Input: part model. Units: mm. Frame: model coordinates. Face numbers are marked on the shaded views. A direction names the side the tool comes from. Round coordinates to 2 decimals unless told otherwise and drop trailing zeros. Loops run counter-clockwise (first coordinate to the right, second up) from the corner with the lowest first, then second, coordinate; pieces in that order, holes last. Notation, with made-up numbers: (25.25, -24.75) -> (62.25, -24.75) arc R9 ccw to (62.25, -15.75) -> close; hole circle Ø5 at (-11, -16). An arc over 180 degrees is marked (long way). Answer as a JSON object with one key per item and string values.
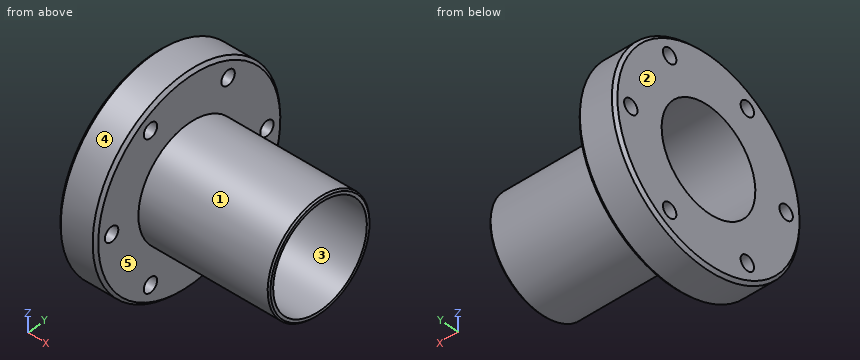
```python
from build123d import *

# Parameters (mm, degrees)
HOLE_WIZARD_M6_1_D       = 5
PATTERN_CIRCULAR_1_COUNT = 6
CHAMFER_1_SIZE           = 1
CHAMFER_2_SIZE           = 1
CHAMFER_3_SIZE           = 0.5


with BuildPart() as part:
    # 스케치1 → 회전1 (revolve)
    with BuildSketch(Plane.XY, mode=Mode.PRIVATE) as revolve_1_sk:
        Polygon((0, 17.5), (0, 35), (13, 35), (13, 19), (58, 19), (58, 17.5), align=None)
    revolve(revolve_1_sk.sketch.rotate(Axis((0, 0, 0), (1, 0, 0)), 90), axis=Axis((0, 0, 0), (1, 0, 0)))

    # M6 나사 구멍1 (through all)
    with Locations(Plane.ZY):
        with Locations((0, 29)):
            hole_wizard_m6_1 = Hole(HOLE_WIZARD_M6_1_D / 2)

    # 원형 패턴1: M6 나사 구멍1 ×6 about axis
    pattern_circular_1_axis = Axis((0, 0, 0), (1, 0, 0))
    for i in range(1, PATTERN_CIRCULAR_1_COUNT):
        add(hole_wizard_m6_1.rotate(pattern_circular_1_axis, i * 360 / PATTERN_CIRCULAR_1_COUNT), mode=Mode.SUBTRACT)

    # 모따기1
    chamfer_1_edges = [part.edges().sort_by_distance(p)[0] for p in [
        (0, 0, -35),
    ]]
    chamfer(chamfer_1_edges, length=CHAMFER_1_SIZE)

    # 모따기2
    chamfer_2_edges = [part.edges().sort_by_distance(p)[0] for p in [
        (13, 0, -35),
    ]]
    chamfer(chamfer_2_edges, length=CHAMFER_2_SIZE)

    # 모따기3
    chamfer_3_edges = [part.edges().sort_by_distance(p)[0] for p in [
        (58, 0, -19),
    ]]
    chamfer(chamfer_3_edges, length=CHAMFER_3_SIZE)


solid = part.part
```
1) Reachability of the marked faces 4 and 5 from +Z, -Z, +X, -X, +Y, -Y: full face, straight path, thin tool, end or side. Return the list, or none.
Output:
{"face 4": "+X, -X", "face 5": "+X"}
2) Ray query, probe 1 along Y at (x, z) = (4, 0); probe 2 along Z at (x, y) = (6, 14); probe 3 along X at (y, z) = (21.5, 10). Return the intervals inside material, ascending.
Output:
{"probe 1": "y = -35 to -31.5, -26.5 to -17.5, 17.5 to 26.5, 31.5 to 35", "probe 2": "z = -32.08 to -27.56, -22.67 to -10.5, 10.5 to 22.67, 27.56 to 32.08", "probe 3": "x = 0 to 13"}
3) Contact query for flat-ended pins moving along their axis: P1, Ø6, axis at x = 38, z = -8, coming from the -Y side; P2, Ø6.5, axis at y = -29, z = 0, coming from the +X side; P3, Ø12, axis at x = 24.5, z = -21, coming from the +Y side. Output: stop coordinate, or through.
Output:
{"P1": "stops at y = -18.33", "P2": "stops at x = 13", "P3": "stops at y = 11.66"}
4) Draft query along Z for the marked faces 1, 2 and 3. Return one class per face: +Z half, -Z half, draft (parallel to the pull), parting line (faces both ways), or undercut.
Output:
{"face 1": "parting line", "face 2": "draft", "face 3": "undercut"}
5) Section D-D, the plane x = 7. Output: boundary loops of the cut face in (y, z).
Output:
{"outline": "circle Ø70 at (0, 0); hole circle Ø5 at (-29, 0); hole circle Ø35 at (0, 0); hole circle Ø5 at (-14.5, -25.11); hole circle Ø5 at (-14.5, 25.11); hole circle Ø5 at (14.5, -25.11); hole circle Ø5 at (14.5, 25.11); hole circle Ø5 at (29, 0)"}
6) Section B-B, the plane z = 0. Output: boundary loops of the cut face in (x, y), plus the area to 3 significant figures.
Output:
{"outline": "(0, -34) -> (1, -35) -> (12, -35) -> (13, -34) -> (13, -31.5) -> (0, -31.5) -> close; (0, -26.5) -> (13, -26.5) -> (13, -19) -> (57.5, -19) -> (58, -18.5) -> (58, -17.5) -> (0, -17.5) -> close; (0, 17.5) -> (58, 17.5) -> (58, 18.5) -> (57.5, 19) -> (13, 19) -> (13, 26.5) -> (0, 26.5) -> close; (0, 31.5) -> (13, 31.5) -> (13, 34) -> (12, 35) -> (1, 35) -> (0, 34) -> close", "area": "458 mm^2"}
7) Section A-A, the plane y = 0. Output: boundary loops of the cut face in (x, z).
Output:
{"outline": "(0, -34) -> (1, -35) -> (12, -35) -> (13, -34) -> (13, -19) -> (57.5, -19) -> (58, -18.5) -> (58, -17.5) -> (0, -17.5) -> close; (0, 17.5) -> (58, 17.5) -> (58, 18.5) -> (57.5, 19) -> (13, 19) -> (13, 34) -> (12, 35) -> (1, 35) -> (0, 34) -> close"}
8) Section C-C, the plane x = 24. Output: boundary loops of the cut face in (y, z).
Output:
{"outline": "circle Ø38 at (0, 0); hole circle Ø35 at (0, 0)"}
